Can you work these out from the drawing? Everything is in mm from the part's minimum corner. A direction names the side the tool comes from. Round coordinates to 2 decimals unless told otherwise and drop trailing zeros. Write each loop counter-clockwise with the first axis right and the second up, starting at its lowest first coordinate (ties: lowest second). Pieces come first, ordered by that corner, then holes. Notation, with made-up numbers: M -28,41.25 L -5,41.25 A3 cw -5,45.25 Z; hole C -6,60.25 d6. An arc over 180 degrees is marked long. Answer in a Markdown table with one row per item. Add a question column.
(1) Suppose I cut it at C-C, the plane z = 27. Write out the boundary of the cut face in (x, y) (1 decimal).
(2) For the marked faces 1 and 2, which set-ups out of +Z, -Z, +X, -X, +Y, -Y let a thin tool reach every point of the face, with its end or its side?
(3) If I drill on probe 1 along Y at (x, z) = (18.25, 14.25); probe 2 along Z at (x, y) = (4, 20.4); probe 3 along Z at (x, y) = (6, 3), over which ranges is the centre line in solid material (lowest first)?
(4) Suppose I cut it at D-D, the plane x = 6. Write out the boundary of the cut face in (y, z).
(5) Suppose I cut it at A-A, the plane x = 4. Write out the boundary of the cut face in (y, z), then the cut area to 3 significant figures.
(6) If we mould it in two halves opening along Y, with no side actions, what happens to the marked faces 3, 4, 5 and 6? For each: released by +Y, released by -Y, zero draft, split by the parting line, or undercut.
(7) Suppose I cut it at B-B, the plane z = 16. Write out the boundary of the cut face in (x, y) (1 decimal).
(8) I'm going to push a flat-ended pin straight in: pin 1 (1.5 mm diameter, centred on x = 11, y = 17, fed in from +Z). Where does the tip first touch, or does it pass through?
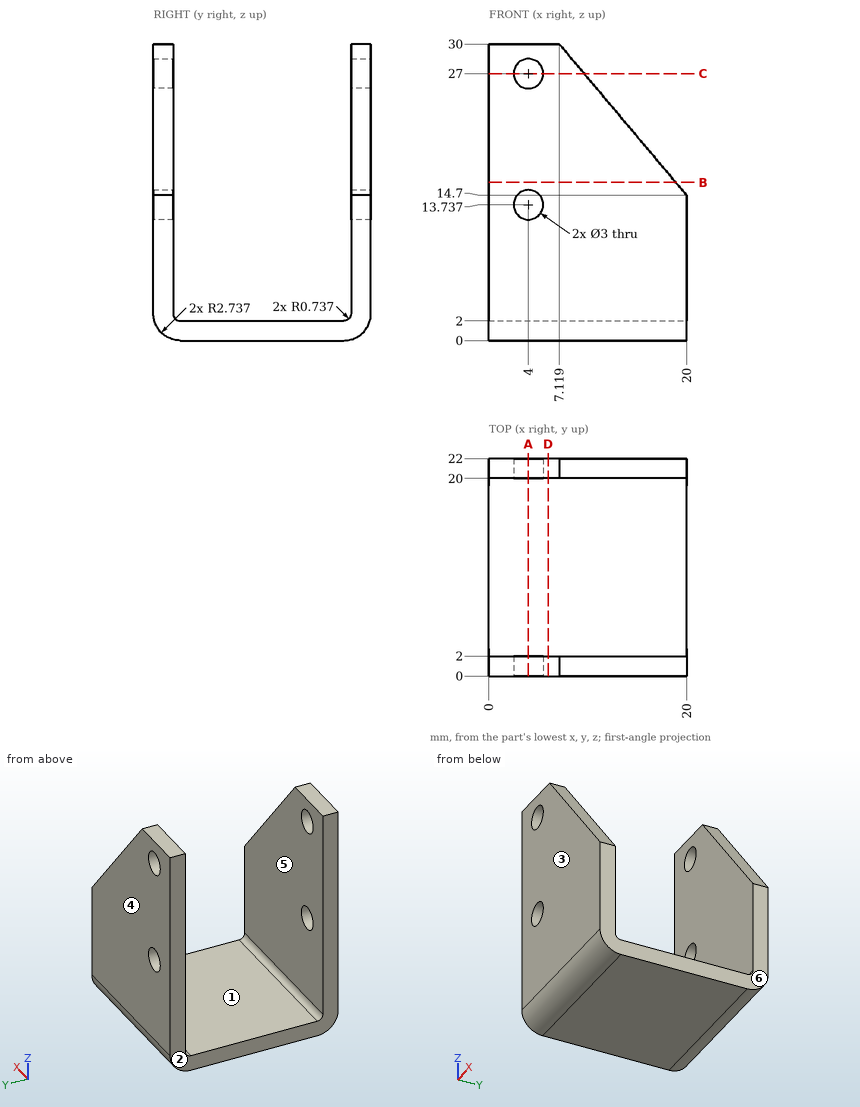
Calculated:
| question | item | result |
|---|---|---|
| 1 | outline | M 0,0 L 2.5,0 L 2.5,2 L 0,2 Z; M 0,20 L 2.5,20 L 2.5,22 L 0,22 Z; M 5.5,0 L 9.6,0 L 9.6,2 L 5.5,2 Z; M 5.5,20 L 9.6,20 L 9.6,22 L 5.5,22 Z |
| 2 | face 1 | +Z, +X, -X |
| 2 | face 2 | +Z, -Z, -X, +Y, -Y |
| 3 | probe 1 | 0 to 2, 20 to 22 |
| 3 | probe 2 | 0.25 to 12.24, 15.24 to 25.5, 28.5 to 30 |
| 3 | probe 3 | 0 to 2 |
| 4 | outline | M 0,2.74 A2.74 ccw 2.74,0 L 19.26,0 A2.74 ccw 22,2.74 L 22,30 L 20,30 L 20,2.74 A0.74 cw 19.26,2 L 2.74,2 A0.74 cw 2,2.74 L 2,30 L 0,30 Z |
| 5 | outline | M 0,2.74 A2.74 ccw 2.74,0 L 19.26,0 A2.74 ccw 22,2.74 L 22,12.24 L 20,12.24 L 20,2.74 A0.74 cw 19.26,2 L 2.74,2 A0.74 cw 2,2.74 L 2,12.24 L 0,12.24 Z; M 0,15.24 L 2,15.24 L 2,25.5 L 0,25.5 Z; M 0,28.5 L 2,28.5 L 2,30 L 0,30 Z; M 20,15.24 L 22,15.24 L 22,25.5 L 20,25.5 Z; M 20,28.5 L 22,28.5 L 22,30 L 20,30 Z |
| 5 | area | 129 mm² |
| 6 | face 3 | released by -Y |
| 6 | face 4 | released by +Y |
| 6 | face 5 | undercut |
| 6 | face 6 | zero draft |
| 7 | outline | M 0,0 L 18.9,0 L 18.9,2 L 0,2 Z; M 0,20 L 18.9,20 L 18.9,22 L 0,22 Z |
| 8 | pin 1 | z = 2 |
